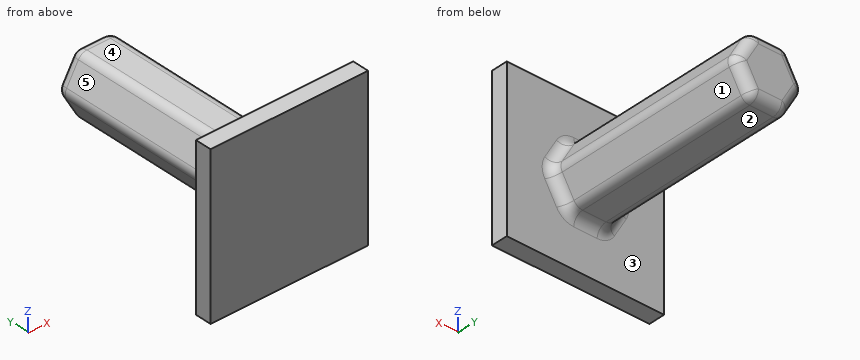
```python
from build123d import *

# Parameters (mm, degrees)
CROQUIS1_W              = 19
CROQUIS1_H              = 19
SALIENTE_EXTRUIR1_DEPTH = 2
SALIENTE_EXTRUIR2_DEPTH = 25
REDONDEO1_R             = 1.2


with BuildPart() as part:
    # Croquis1 → Saliente-Extruir1 (new body)
    with BuildSketch(Plane(origin=(0, 0, 0), x_dir=(1, 0, 0), z_dir=(0, 1, 0))):
        Rectangle(CROQUIS1_W, CROQUIS1_H)
    extrude(amount=SALIENTE_EXTRUIR1_DEPTH)

    # Croquis2 → Saliente-Extruir2 (add)
    with BuildSketch(Plane(origin=(0, 2, 0), x_dir=(1, 0, 0), z_dir=(0, 1, 0))):
        Polygon((4.214656965, 0), (2.107328483, 3.65), (-2.107328483, 3.65), (-4.214656965, 0), (-2.107328483, -3.65), (2.107328483, -3.65), align=None)
    extrude(amount=SALIENTE_EXTRUIR2_DEPTH)

    # Redondeo1
    redondeo1_edges = [part.edges().sort_by_distance(p)[0] for p in [
        (3.160992724, 2, 1.825),
        (2.107328483, 14.5, 3.65),
        (3.160992724, 2, -1.825),
        (4.214656965, 14.5, 0),
        (0, 2, -3.65),
        (2.107328483, 14.5, -3.65),
        (-3.160992724, 2, -1.825),
        (-2.107328483, 14.5, -3.65),
        (-3.160992724, 2, 1.825),
        (-4.214656965, 14.5, 0),
        (0, 2, 3.65),
        (-2.107328483, 14.5, 3.65),
        (3.160992724, 27, 1.825),
        (3.160992724, 27, -1.825),
        (0, 27, -3.65),
        (-3.160992724, 27, -1.825),
        (-3.160992724, 27, 1.825),
        (0, 27, 3.65),
    ]]
    fillet(redondeo1_edges, radius=REDONDEO1_R)


solid = part.part
```
Design review of the part built by this model. Coordinates are the model's own, in mm. Face numbers are marked on the shaded views. A direction names the side the tool comes from. Round coordinates to 2 decimals unless told otherwise and drop trailing zeros. Write each loop counter-clockwise with the first axis right and the second up, starting at its lowest first coordinate (ties: lowest second). Pieces come first, ordered by that corner, then holes. Notation, with made-up numbers: (65, -22.5) -> (87, -22.5) arc R37 ccw to (87, 14.5) -> close; hole circle Ø2 at (78, 21.5). An arc over 180 degrees is marked (long way). Write item = value, one per line. Start each with the question number.
1) Take a section at A-A, the plane y = 16.25. State the section outline as (x, z) points.
2) Take a section at C-C, the plane z = 7. State the section outline as (x, y) points.
3) Clearance check with flat-ended pins moving along their axes: pin 1 (8 mm diameter, centred on y = 12.5, z = 2.5, fed in from +X); pin 2 (1.4 mm diameter, centred on x = 0.5, y = 14, fed in from -Z); pin 3 (4 mm diameter, centred on x = 1, z = -6.5, fed in from +Y). State where each tip first meets the part, or that it passes through.
4) Wall thickness on probe 1 along Y at (x, z) = (-2.5, 7.75); probe 2 along Y at (x, z) = (3.5, -1.75); probe 3 along Z at (x, y) = (-0.5, 22.25): over which ranges is each line inside the solid? List them lowest first. Write a range as from..to.
5) Take a section at B-B, the plane x = -0.5. State the section outline as (y, z) points, plus the area to 4 significant figures.
6) Take a section at D-D, the plane x = -7. State the section outline as (y, z) points, plus the area to 3 significant figures.
7) Tool access review of the marked faces 1, 2, 3, 4 and 5: name each direction out of +Z, -Z, +X, -X, +Y, -Y from which nothing blocks a thin tool from reaching the whole face with its end or side.
Results list:
q1.outline = (-3.87, -0.6) -> (-2.45, -3.05) arc R1.2 ccw to (-1.41, -3.65) -> (1.41, -3.65) arc R1.2 ccw to (2.45, -3.05) -> (3.87, -0.6) arc R1.2 ccw to (3.87, 0.6) -> (2.45, 3.05) arc R1.2 ccw to (1.41, 3.65) -> (-1.41, 3.65) arc R1.2 ccw to (-2.45, 3.05) -> (-3.87, 0.6) arc R1.2 ccw to start
q2.outline = (-9.5, 0) -> (9.5, 0) -> (9.5, 2) -> (-9.5, 2) -> close
q3.pin_1 = 4.03
q3.pin_2 = -3.65
q3.pin_3 = 2.05
q4.probe_1 = 0..2
q4.probe_2 = 0..2.46
q4.probe_3 = -3.65..3.65
q5.outline = (0, -9.5) -> (2, -9.5) -> (2, -4.85) arc R1.2 cw to (3.2, -3.65) -> (25.8, -3.65) arc R1.2 ccw to (27, -2.45) -> (27, 2.45) arc R1.2 ccw to (25.8, 3.65) -> (3.2, 3.65) arc R1.2 cw to (2, 4.85) -> (2, 9.5) -> (0, 9.5) -> close
q5.area = 220.5 mm²
q6.outline = (0, -9.5) -> (2, -9.5) -> (2, 9.5) -> (0, 9.5) -> close
q6.area = 38.0 mm²
q7.face_1 = -Z, +X, +Y
q7.face_2 = -Z, +X, -X, +Y
q7.face_3 = +Y
q7.face_4 = +Z, +X, -X, +Y
q7.face_5 = +Z, -X, +Y
